Design review of the part built by this model. Coordinates are the model's own, in mm. Round coordinates to 2 decimals unless told otherwise and drop trailing zeros. Write item = value, one per line.
from build123d import *

# Parameters (mm, degrees)
BOSS_EXTRUDE1_DEPTH = 4


with BuildPart() as part:
    # Sketch2 → Boss-Extrude1 (new body)
    with BuildSketch(Plane.XY):
        Polygon((-778.491602678, 45.210025961), (-778.491602678, 41.210025961), (-774.491602678, 41.210025961), (-774.491602678, 1.805025961), (-750.491602678, 1.805025961), (-756.491602678, 9.805025961), (-732.491602678, 9.805025961), (-738.491602678, 1.805025961), (-714.491602678, 1.805025961), (-720.491602678, 9.805025961), (-696.491602678, 9.805025961), (-702.491602678, 1.805025961), (-678.491602678, 1.805025961), (-678.491602678, 41.210025961), (-674.491602678, 41.210025961), (-674.491602678, 1.805025961), (-650.491602678, 1.805025961), (-656.491602678, 9.805025961), (-632.491602678, 9.805025961), (-638.491602678, 1.805025961), (-614.491602678, 1.805025961), (-620.491602678, 9.805025961), (-596.491602678, 9.805025961), (-602.491602678, 1.805025961), (-578.491602678, 1.805025961), (-578.491602678, 41.210025961), (-574.491602678, 41.210025961), (-574.491602678, 1.805025961), (-550.491602678, 1.805025961), (-556.491602678, 9.805025961), (-532.491602678, 9.805025961), (-538.491602678, 1.805025961), (-514.491602678, 1.805025961), (-520.491602678, 9.805025961), (-496.491602678, 9.805025961), (-502.491602678, 1.805025961), (-478.491602678, 1.805025961), (-478.491602678, 41.210025961), (-474.491602678, 41.210025961), (-474.491602678, 1.805025961), (-450.491602678, 1.805025961), (-456.491602678, 9.805025961), (-432.491602678, 9.805025961), (-438.491602678, 1.805025961), (-414.491602678, 1.805025961), (-420.491602678, 9.805025961), (-396.491602678, 9.805025961), (-402.491602678, 1.805025961), (-378.491602678, 1.805025961), (-378.491602678, 41.210025961), (-374.491602678, 41.210025961), (-374.491602678, 1.805025961), (-350.491602678, 1.805025961), (-356.491602678, 9.805025961), (-332.491602678, 9.805025961), (-338.491602678, 1.805025961), (-314.491602678, 1.805025961), (-320.491602678, 9.805025961), (-296.491602678, 9.805025961), (-302.491602678, 1.805025961), (-278.491602678, 1.805025961), (-278.491602678, 41.210025961), (-274.491602678, 41.210025961), (-274.491602678, 1.805025961), (-250.491602678, 1.805025961), (-256.491602678, 9.805025961), (-232.491602678, 9.805025961), (-238.491602678, 1.805025961), (-214.491602678, 1.805025961), (-220.491602678, 9.805025961), (-196.491602678, 9.805025961), (-202.491602678, 1.805025961), (-178.491602678, 1.805025961), (-178.491602678, 41.210025961), (-174.491602678, 41.210025961), (-174.491602678, 1.805025961), (-150.491602678, 1.805025961), (-156.491602678, 9.805025961), (-132.491602678, 9.805025961), (-138.491602678, 1.805025961), (-114.491602678, 1.805025961), (-120.491602678, 9.805025961), (-96.491602678, 9.805025961), (-102.491602678, 1.805025961), (-78.491602678, 1.805025961), (-78.491602678, 41.210025961), (-74.491602678, 41.210025961), (-74.491602678, 1.805025961), (-50.491602678, 1.805025961), (-56.491602678, 9.805025961), (-32.491602678, 9.805025961), (-38.491602678, 1.805025961), (-14.491602678, 1.805025961), (-20.491602678, 9.805025961), (3.508397322, 9.805025961), (-2.491602678, 1.805025961), (21.508397322, 1.805025961), (21.508397322, 41.210025961), (25.508397322, 41.210025961), (25.508397322, 1.805025961), (49.508397322, 1.805025961), (43.508397322, 9.805025961), (67.508397322, 9.805025961), (61.508397322, 1.805025961), (85.508397322, 1.805025961), (79.508397322, 9.805025961), (103.508397322, 9.805025961), (97.508397322, 1.805025961), (121.508397322, 1.805025961), (121.508397322, 41.210025961), (125.508397322, 41.210025961), (125.508397322, 1.805025961), (149.508397322, 1.805025961), (143.508397322, 9.805025961), (167.508397322, 9.805025961), (161.508397322, 1.805025961), (185.508397322, 1.805025961), (179.508397322, 9.805025961), (203.508397322, 9.805025961), (197.508397322, 1.805025961), (221.508397322, 1.805025961), (221.508397322, 41.210025961), (225.508397322, 41.210025961), (225.508397322, 1.805025961), (249.508397322, 1.805025961), (243.508397322, 9.805025961), (267.508397322, 9.805025961), (261.508397322, 1.805025961), (285.508397322, 1.805025961), (279.508397322, 9.805025961), (303.508397322, 9.805025961), (297.508397322, 1.805025961), (321.508397322, 1.805025961), (321.508397322, 41.210025961), (325.508397322, 41.210025961), (325.508397322, 1.805025961), (349.508397322, 1.805025961), (343.508397322, 9.805025961), (367.508397322, 9.805025961), (361.508397322, 1.805025961), (385.508397322, 1.805025961), (379.508397322, 9.805025961), (403.508397322, 9.805025961), (397.508397322, 1.805025961), (421.508397322, 1.805025961), (421.508397322, 41.210025961), (425.508397322, 41.210025961), (425.508397322, 1.805025961), (449.508397322, 1.805025961), (443.508397322, 9.805025961), (467.508397322, 9.805025961), (461.508397322, 1.805025961), (485.508397322, 1.805025961), (479.508397322, 9.805025961), (503.508397322, 9.805025961), (497.508397322, 1.805025961), (521.508397322, 1.805025961), (521.508397322, 41.210025961), (525.508397322, 41.210025961), (525.508397322, 1.805025961), (549.508397322, 1.805025961), (543.508397322, 9.805025961), (567.508397322, 9.805025961), (561.508397322, 1.805025961), (585.508397322, 1.805025961), (579.508397322, 9.805025961), (603.508397322, 9.805025961), (597.508397322, 1.805025961), (621.508397322, 1.805025961), (621.508397322, 41.210025961), (625.508397322, 41.210025961), (625.508397322, 1.805025961), (649.508397322, 1.805025961), (643.508397322, 9.805025961), (667.508397322, 9.805025961), (661.508397322, 1.805025961), (685.508397322, 1.805025961), (679.508397322, 9.805025961), (703.508397322, 9.805025961), (697.508397322, 1.805025961), (721.508397322, 1.805025961), (721.508397322, 41.210025961), (725.508397322, 41.210025961), (725.508397322, 45.210025961), align=None)
    extrude(amount=BOSS_EXTRUDE1_DEPTH)


solid = part.part
Item 1: Take a section at A-A, the plane y = 25. Count the separate pieces of the cut face and the enclosed holes in it, and give its area (3 significant figures).
Data:
separate_pieces = 15
enclosed_holes = 0
area = 5,760 mm2
Item 2: Insertion check: P1, Ø2, axis at x = 492.5, z = 2, coming from the -Y side (3 decimals); P2, Ø2, axis at y = 14.5, z = 2.5, coming from the -X side; P3, Ø1.2, axis at y = 16, z = 2.5, coming from the +X side. Each pin has a flat end and moves straight along its axis. Give the tip position at first contact, or say it passes through.
Data:
P1 = 9.805
P2 = -774.49
P3 = 721.51
Item 3: For line 1 along Y through (x, z) = (-708, 3.7); line 2 along Y through (x, z) = (-517, 1.7); line 3 along Y through (x, z) = (-538, 1.55), list the stretches that pass through material, from the lowest coordinate up. Write a range as [from, to].
Data:
line_1 = [9.81, 45.21]
line_2 = [1.81, 5.15], [9.81, 45.21]
line_3 = [1.81, 2.46], [9.81, 45.21]
